Source: CAD feature listing. Evaluate the final solid. Frame: model axes, mm. A direction names the side the tool comes from. Round coordinates to 2 decimals unless told otherwise and drop trailing zeros. Loops run counter-clockwise (first coordinate to the right, second up) from the corner with the lowest first, then second, coordinate; pieces in that order, holes last. Notation, with made-up numbers: M -28,74 L -19,74 A19 cw -19,102 Z; hole C -29,60.5 d10. An arc over 180 degrees is marked long. One line per item, written item: value.
from build123d import *

# Parameters (mm, degrees)
SKETCH1_W                 = 125
SKETCH1_H                 = 26
BOSS_EXTRUDE1_DEPTH       = 10
SKETCH2_W                 = 25
SKETCH2_H                 = 26
BOSS_EXTRUDE2_DEPTH       = 27.5
FILLET3_R                 = 5
FILLET4_R                 = 3
SKETCH3_W                 = 40
SKETCH3_H                 = 20
CUT_EXTRUDE2_DEPTH        = 2
SKETCH5_W                 = 40
SKETCH5_H                 = 20
CUT_EXTRUDE3_DEPTH        = 2
SKETCH6_R                 = 11
CUT_EXTRUDE5_DEPTH        = 7
SKETCH7_R                 = 11
CUT_EXTRUDE6_DEPTH        = 7
SKETCH8_W                 = 25
SKETCH8_H                 = 26
CUT_EXTRUDE7_DEPTH        = 2
SKETCH9_W                 = 40
SKETCH9_H                 = 20
CUT_EXTRUDE8_DEPTH        = 1
F_1_5MM_DOWEL_HOLE1_D     = 1.5
F_1_5MM_DOWEL_HOLE1_DEPTH = 8
F_1_5MM_DOWEL_HOLE1_TIP   = 0.450645464


with BuildPart() as part:
    # Sketch1 → Boss-Extrude1 (new body)
    with BuildSketch(Plane(origin=(0, 0, 0), x_dir=(1, 0, 0), z_dir=(0, 1, 0))):
        with Locations((62.5, 13)):
            Rectangle(SKETCH1_W, SKETCH1_H)
    extrude(amount=BOSS_EXTRUDE1_DEPTH)

    # Sketch2 → Boss-Extrude2 (add)
    with BuildSketch(Plane(origin=(0, 10, 0), x_dir=(1, 0, 0), z_dir=(0, 1, 0))):
        with Locations((62.5, 13)):
            Rectangle(SKETCH2_W, SKETCH2_H)
    extrude(amount=BOSS_EXTRUDE2_DEPTH)

    # Fillet3
    fillet3_edges = [part.edges().sort_by_distance(p)[0] for p in [
        (0, 5, -26),
        (125, 5, -26),
        (125, 5, 0),
        (0, 5, 0),
    ]]
    fillet(fillet3_edges, radius=FILLET3_R)

    # Fillet4
    fillet4_edges = [part.edges().sort_by_distance(p)[0] for p in [
        (62.5, 0, 0),
        (0, 0, -13),
        (62.5, 0, -26),
        (125, 0, -13),
        (123.535533906, 0, -1.464466094),
        (123.535533906, 0, -24.535533906),
        (1.464466094, 0, -24.535533906),
        (1.464466094, 0, -1.464466094),
    ]]
    fillet(fillet4_edges, radius=FILLET4_R)

    # Sketch3 → Cut-Extrude2 (cut)
    with BuildSketch(Plane(origin=(0, 10, 0), x_dir=(1, 0, 0), z_dir=(0, 1, 0))):
        with Locations((30, 13)):
            Rectangle(SKETCH3_W, SKETCH3_H)
    extrude(amount=-CUT_EXTRUDE2_DEPTH, mode=Mode.SUBTRACT)

    # Sketch5 → Cut-Extrude3 (cut)
    with BuildSketch(Plane(origin=(0, 10, 0), x_dir=(1, 0, 0), z_dir=(0, 1, 0))):
        with Locations((95, 13)):
            Rectangle(SKETCH5_W, SKETCH5_H)
    extrude(amount=-CUT_EXTRUDE3_DEPTH, mode=Mode.SUBTRACT)

    # Sketch6 → Cut-Extrude5 (cut)
    with BuildSketch(Plane(origin=(0, 0, 0), x_dir=(-1, 0, 0), z_dir=(0, -1, 0))):
        with Locations(Location((-19, 13, 0), (0, 0, 90))):
            Circle(SKETCH6_R)
    extrude(amount=-CUT_EXTRUDE5_DEPTH, mode=Mode.SUBTRACT)

    # Sketch7 → Cut-Extrude6 (cut)
    with BuildSketch(Plane(origin=(0, 0, 0), x_dir=(-1, 0, 0), z_dir=(0, -1, 0))):
        with Locations(Location((-106, 13, 0), (0, 0, 90))):
            Circle(SKETCH7_R)
    extrude(amount=-CUT_EXTRUDE6_DEPTH, mode=Mode.SUBTRACT)

    # Sketch8 → Cut-Extrude7 (cut)
    with BuildSketch(Plane(origin=(0, 37.5, 0), x_dir=(1, 0, 0), z_dir=(0, 1, 0))):
        with Locations((62.5, 13)):
            Rectangle(SKETCH8_W, SKETCH8_H)
    extrude(amount=-CUT_EXTRUDE7_DEPTH, mode=Mode.SUBTRACT)

    # Sketch9 → Cut-Extrude8 (cut)
    with BuildSketch(Plane(origin=(0, 8, 0), x_dir=(1, 0, 0), z_dir=(0, 1, 0))):
        with Locations((30, 13)):
            Rectangle(SKETCH9_W, SKETCH9_H)
        with Locations((95, 13)):
            Rectangle(SKETCH9_W, SKETCH9_H)
    extrude(amount=-CUT_EXTRUDE8_DEPTH, mode=Mode.SUBTRACT)

    # Ø1.5mm Dowel Hole1
    with Locations(Plane(origin=(54.9, 35.5, -18), x_dir=(0, 0, 1), z_dir=(0, 1, 0))):
        with Locations((0, 0), (0, 15.2), (10, 15.2), (10, 0)):
            Hole(F_1_5MM_DOWEL_HOLE1_D / 2, depth=F_1_5MM_DOWEL_HOLE1_DEPTH)
            with Locations((0, 0, -(F_1_5MM_DOWEL_HOLE1_DEPTH + F_1_5MM_DOWEL_HOLE1_TIP / 2))):  # 118° drill point
                Cone(0, F_1_5MM_DOWEL_HOLE1_D / 2, F_1_5MM_DOWEL_HOLE1_TIP, mode=Mode.SUBTRACT)


solid = part.part
1. Section query D-D (y = 18). Return the cut outline in (x, z), and give its area (3 significant figures).
Report:
outline: M 50,-26 L 75,-26 L 75,0 L 50,0 Z
area: 650 mm2
2. Pull-direction query (X, two-part tool) for faces 4 (the face through (40, 7, -13)), 5 (the face through (123, 7, -25)), 6 (the face through (11, 7, -4)), 7 (the face through (63.3, 0.86, -0.9)); classes: released by +X, released by -X, zero draft, split by the parting line, or undercut.
Report:
face 4: undercut
face 5: released by +X
face 6: undercut
face 7: zero draft
3. Reachability of faces 1 (the face through (116, 10, -13)), 2 (the face through (125, 6, -13)), 3 (the face through (95, 9, -23)) from +Z, -Z, +X, -X, +Y, -Y: full face, straight path, thin tool, end or side. Return the list, or none.
Report:
face 1: +Z, -Z, +X, +Y
face 2: +Z, -Z, +X, +Y, -Y
face 3: +Y
4. Section query C-C (x = 19). Return the cut outline in (y, z), and give its area (3 significant figures).
Report:
outline: M 0.17,-24 A3 ccw 3,-26 L 10,-26 L 10,-23 L 7,-23 L 7,-24 Z; M 0.17,-2 L 7,-2 L 7,-3 L 10,-3 L 10,0 L 3,0 A3 ccw Z
area: 42.3 mm2
5. Ray query, line 1 (X direction, y = 30.5, z = -8); line 2 (X direction, y = 9.5, z = -13); line 3 (Z direction, x = 54.9, y = 30.25). Return the intervals inside material, ascending. Write a range as [from, to].
Report:
line 1: x = [50, 54.15], [55.65, 69.35], [70.85, 75]
line 2: x = [0, 10], [50, 75], [115, 125]
line 3: z = [-26, -18.75], [-17.25, -8.75], [-7.25, 0]
6. Section query B-B (x = 35.5). Return the cut outline in (y, z).
Report:
outline: M 0,-23 A3 ccw 3,-26 L 10,-26 L 10,-23 L 7,-23 L 7,-3 L 10,-3 L 10,0 L 3,0 A3 ccw 0,-3 Z
7. Section query A-A (y = 5). Return the cut outline in (x, z).
Report:
outline: M 0,-21 A5 ccw 5,-26 L 120,-26 A5 ccw 125,-21 L 125,-5 A5 ccw 120,0 L 5,0 A5 ccw 0,-5 Z; hole C 19,-13 d22; hole C 106,-13 d22
8. Pin query (flat end, axial travel): pin 1 (12 mm diameter, centred on y = 26.5, z = -18.5, fed in from -X); pin 2 (2 mm diameter, centred on x = 43.5, z = -4.5, fed in from +Y); pin 3 (1.4 mm diameter, centred on x = 70.1, z = -8, fed in from +Y). Return the tip coordinate at first contact, or that it passes through.
Report:
pin 1: stops at x = 50
pin 2: stops at y = 7
pin 3: stops at y = 27.47
